```python
from build123d import *

# Parameters (mm, degrees)
FILLET001_R       = 3
BOX005_W          = 10.4
BOX005_H          = 5.2
BOX005_DEPTH      = 5.2
BOX006_W          = 16
BOX006_H          = 16
BOX006_DEPTH      = 8
CYLINDER009_R     = 5.2
CYLINDER009_DEPTH = 10.2
CYLINDER010_R     = 2
CYLINDER010_DEPTH = 8


with BuildPart() as part:
    # Cone → Cone (revolve)
    with BuildSketch(Plane.XZ):
        Polygon((0, 0), (14, 0), (9, 10), (0, 10), align=None)
    revolve(axis=Axis((0, 0, 0), (0, 0, 1)))

    # Fillet001
    fillet001_edges = [part.edges().sort_by_distance(p)[0] for p in [
        (-9, 0, 10),
    ]]
    fillet(fillet001_edges, radius=FILLET001_R)

    # Box005 → Box005 (cut)
    with BuildSketch(Plane(origin=(-5.2, -5.2, 4.8), x_dir=(1, 0, 0), z_dir=(0, 0, 1))):
        with Locations((5.2, 2.6)):
            Rectangle(BOX005_W, BOX005_H)
    extrude(amount=BOX005_DEPTH, mode=Mode.SUBTRACT)

    # Box006 → Box006 (join)
    with BuildSketch(Plane(origin=(-8, -8, -8), x_dir=(1, 0, 0), z_dir=(0, 0, 1))):
        with Locations((8, 8)):
            Rectangle(BOX006_W, BOX006_H)
    extrude(amount=BOX006_DEPTH)

    # Cylinder009 → Cylinder009 (cut)
    with BuildSketch(Plane.XY.offset(-0.2)):
        Circle(CYLINDER009_R)
    extrude(amount=CYLINDER009_DEPTH, mode=Mode.SUBTRACT)

    # Cylinder010 → Cylinder010 (cut)
    with BuildSketch(Plane.XY.offset(-8)):
        Circle(CYLINDER010_R)
    extrude(amount=CYLINDER010_DEPTH, mode=Mode.SUBTRACT)


with BuildPart() as part_1:
    # Body005 placement: moved
    add(part.part.moved(Location((1, -43, -192))))


solid = part_1.part
```
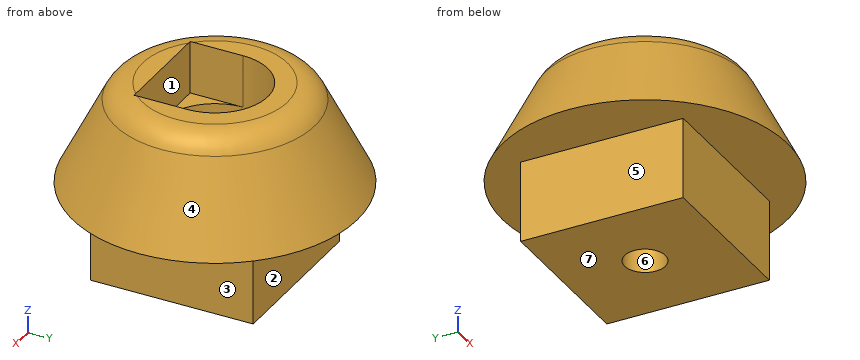
Could you check a few things on this model? Use its own coordinates, in mm. Face numbers are marked on the shaded views. A direction names the side the tool comes from. Round coordinates to 2 decimals unless told otherwise and drop trailing zeros. Loops run counter-clockwise (first coordinate to the right, second up) from the corner with the lowest first, then second, coordinate; pieces in that order, holes last.
Q1. Please list where these lines run through material, in increasing order: L1, parallel to Y at x = 1, z = -194.5; L2, parallel to X at y = -43, z = -197.5; L3, parallel to Z at x = 0, y = -46.5.
Q2. I want a section at B-B (z = -191). Write out the boundary of the cut face in (x, y), and give its area (3 significant figures).
Q3. For P1, Ø6.5, axis at y = -42.5, z = -194.5, coming from the -X side; P2, Ø10, axis at x = -3, z = -186, coming from the -Y side; P3, Ø3.5, axis at x = 1, y = -43, coming from the +Z side; P4, Ø1.5, axis at y = -45, z = -188, coming from the +X side, each with a flat end and sliding along its axis, tell me the tip position at first contact or that it passes through.
Q4. On a 3-axis mill with a long thin cutter (end or side, diameter ignored), from which of +Z, -Z, +X, -X, +Y, -Y can I reach the whole of each face in a straight line? I mean the marked faces 1, 2 and 3. Say none if no direction works.
Q5. I want a section at A-A (z = -194.25). Write out the boundary of the cut face in (x, y).
Q6. Thinking about a two-plate mould opening in X: for the marked faces 4, 5, 6 and 7, which applies, pulls with the +X half, pulls with the -X half, needs draft (parallel to the pull), parting line crosses it, or undercut?
Answer below:
1. L1: y = -51 to -45, -41 to -35
1. L2: x = -7 to -1, 3 to 9
1. L3: z = -200 to -192.2
2. outline: circle Ø27 at (1, -43); hole circle Ø10.4 at (1, -43)
2. area: 488 mm2
3. P1: stops at x = -13
3. P2: stops at y = -56.15
3. P3: passes through
3. P4: stops at x = 13.23
4. face 1: +Z
4. face 2: -Z, +X, -X, +Y
4. face 3: -Z, +X, +Y, -Y
5. outline: (-7, -51) - (9, -51) - (9, -35) - (-7, -35) - close; hole circle Ø4 at (1, -43)
6. face 4: parting line crosses it
6. face 5: pulls with the -X half
6. face 6: undercut
6. face 7: needs draft
